Here's how the part is built. I have some questions about the finished solid (model axes, mm). A direction names the side the tool comes from. Coordinates: 2 decimals unless noted, no trailing zeros. Use a Markdown table: item, result. Add a question column.
Item 1: On a 3-axis mill with a long thin cutter (end or side, diameter ignored), from which of +Z, -Z, +X, -X, +Y, -Y can I reach the whole of each face in a straight line? I mean faces 5 (the cylindrical face through (3.04, -25.75, 0.06)), 6 (the conical face through (12.865, 0.153, -40.634)), 7 (the flat face through (7, 7, -30)), 8 (the flat face through (10, 15, -19)). Say none if no direction works.
Item 2: If we mould it in two halves opening along Z, with no side actions, what happens to faces 1 (the cylindrical face through (3.04, -0.12, -21.75)), 2 (the cylindrical face through (3.04, 25.75, -0.06)), 3 (the cylindrical face through (3.042, -19.696, 9.226)), 4 (the cylindrical face through (4.93, 12.25, -17.76))? For each: pulls with the +Z half, pulls with the -Z half, needs draft (parallel to the pull), parting line crosses it, or undercut.
Item 3: Imagine slicing it at A-A, the plane y = 0. Count the separate pieces of the cut face and the enclosed holes in it, and give its area (3 significant figures).
Item 4: If I drill on line 1 along Z through (x, y) = (6.75, -0.5); line 2 along Y through (x, z) = (4.75, 0); line 3 along X through (y, z) = (10, 22), over which ranges is the centre line in solid material (lowest first)? Write a range as from..to.
Item 5: Will these pins go through, and if not, where does the flat tip stop? pin 1 Ø9 at (y, z) = (-16, 18) entering from +X; pin 2 Ø10.5 at (y, z) = (0, -30) entering from +X; pin 3 Ø2.5 at (y, z) = (22, 0.5) entering from +X; pin 4 Ø9 at (y, z) = (0, -30) entering from -X.
```python
from build123d import *

# Parameters (mm, degrees)
SKETCH_1_R               = 26.5
SKETCH_1_R_2             = 16.5
EXTRUDE_1_DEPTH          = 6
SKETCH_2_R               = 2.05
CUT_EXTRUDE_1_DEPTH      = 10
PATTERN_CIRCULAR_1_COUNT = 3
PATTERN_CIRCULAR_1_ANGLE = 100
SKETCH_3_R               = 2.05
SKETCH_3_R_2             = 2.6
SKETCH_3_R_3             = 16.5
EXTRUDE_2_DEPTH          = 7
CUT_EXTRUDE_START        = -6
CUT_EXTRUDE_2_OUTLINE_R  = 26.5
CUT_EXTRUDE_2_DEPTH      = 6
CHAMFER_1_SIZE           = 1
FILLET_1_R               = 5
SKETCH_5_R               = 4.075
SKETCH_5_R_2             = 4
CUT_EXTRUDE_3_DEPTH      = 3
PATTERN_CIRCULAR_2_COUNT = 2
PATTERN_CIRCULAR_2_ANGLE = 50
F_2_THE_OTHER_WAY_COUNT  = 2
F_2_THE_OTHER_WAY_ANGLE  = 50
SKETCH_6_R               = 6.6
CUT_EXTRUDE_4_DEPTH      = 4
SKETCH_7_R               = 7.6
CUT_EXTRUDE_5_DEPTH      = 1
SKETCH_8_R               = 6.15
CUT_EXTRUDE_6_DEPTH      = 2
CHAMFER_2_SIZE           = 0.5


# Read off the part's stored shape, not the designer's step: 切除-拉伸2
with BuildPart() as part:
    # 草图1 → 凸台-拉伸1 (new body)
    with BuildSketch(Plane(origin=(0, 0, 0), x_dir=(0, 0, -1), z_dir=(1, 0, 0))):
        Circle(SKETCH_1_R)
        Circle(SKETCH_1_R_2, mode=Mode.SUBTRACT)
    extrude(amount=EXTRUDE_1_DEPTH)

    # 草图2 → 切除-拉伸1 (cut)
    with BuildSketch(Plane.ZY):
        with Locations((16.661466638, 13.980630511)):
            Circle(SKETCH_2_R)
        with Locations((-16.661466638, -13.980630511)):
            Circle(SKETCH_2_R)
    cut_extrude_1 = extrude(amount=-CUT_EXTRUDE_1_DEPTH, mode=Mode.SUBTRACT)

    # 阵列(圆周)1: 切除-拉伸1 ×3 about axis
    pattern_circular_1_axis = Axis((0, 0, 0), (-1, 0, 0))
    for i in range(1, PATTERN_CIRCULAR_1_COUNT):
        add(cut_extrude_1.rotate(pattern_circular_1_axis, i * PATTERN_CIRCULAR_1_ANGLE / (PATTERN_CIRCULAR_1_COUNT - 1)), mode=Mode.SUBTRACT)

    # 草图3 → 凸台-拉伸2 (add)
    with BuildSketch(Plane.ZY.offset(-6)):
        with BuildLine():
            ThreePointArc((-35.683333333, 9.418052995), (-41, 0), (-35.683333333, -9.418052995))
            Line((-35.683333333, -9.418052995), (-13.691666667, -22.688945852))
            ThreePointArc((-13.691666667, -22.688945852), (26.5, 0), (-13.691666667, 22.688945852))
            Line((-13.691666667, 22.688945852), (-35.683333333, 9.418052995))
        make_face()
        with Locations((-16.661466638, -13.980630511)):
            Circle(SKETCH_3_R, mode=Mode.SUBTRACT)
        with Locations(Location((0, -21.75, 0), (0, 0, 50))):
            Circle(SKETCH_3_R, mode=Mode.SUBTRACT)
        with Locations(Location((16.661466638, -13.980630511, 0), (0, 0, 100))):
            Circle(SKETCH_3_R, mode=Mode.SUBTRACT)
        with Locations(Location((-30, 0, 0), (0, 0, 180))):
            Circle(SKETCH_3_R_2, mode=Mode.SUBTRACT)
        with Locations(Location((-16.661466638, 13.980630511, 0), (0, 0, 100))):
            Circle(SKETCH_3_R, mode=Mode.SUBTRACT)
        with Locations(Location((0, 0, 0), (0, 0, 180))):
            Circle(SKETCH_3_R_3, mode=Mode.SUBTRACT)
        with Locations(Location((0, 21.75, 0), (0, 0, 50))):
            Circle(SKETCH_3_R, mode=Mode.SUBTRACT)
        with Locations((16.661466638, 13.980630511)):
            Circle(SKETCH_3_R, mode=Mode.SUBTRACT)
    extrude(amount=-EXTRUDE_2_DEPTH)

    # 切除-拉伸2 outline → 切除-拉伸2 (cut)
    with BuildSketch(Plane.ZY.offset(CUT_EXTRUDE_START)):
        Circle(CUT_EXTRUDE_2_OUTLINE_R)
        with BuildLine():
            ThreePointArc((-18.939960291, -10.693007255), (-21.75, 0), (-18.939960291, 10.693007255))
            ThreePointArc((-18.939960291, 10.693007255), (-19.72564441, 16.551780949), (-13.819446038, 16.795398513))
            ThreePointArc((-13.819446038, 16.795398513), (-9.191947193, 19.712194368), (-3.983053015, 21.382183908))
            ThreePointArc((-3.983053015, 21.382183908), (0, 25.75), (3.983053015, 21.382183908))
            ThreePointArc((3.983053015, 21.382183908), (9.191947193, 19.712194368), (13.819446038, 16.795398513))
            ThreePointArc((13.819446038, 16.795398513), (19.72564441, 16.551780949), (18.939960291, 10.693007255))
            ThreePointArc((18.939960291, 10.693007255), (21.75, 0), (18.939960291, -10.693007255))
            ThreePointArc((18.939960291, -10.693007255), (19.72564441, -16.551780949), (13.819446038, -16.795398513))
            ThreePointArc((13.819446038, -16.795398513), (9.191947193, -19.712194368), (3.983053015, -21.382183908))
            ThreePointArc((3.983053015, -21.382183908), (0, -25.75), (-3.983053015, -21.382183908))
            ThreePointArc((-3.983053015, -21.382183908), (-9.191947193, -19.712194368), (-13.819446038, -16.795398513))
            ThreePointArc((-13.819446038, -16.795398513), (-19.72564441, -16.551780949), (-18.939960291, -10.693007255))
        make_face(mode=Mode.SUBTRACT)
    extrude(amount=CUT_EXTRUDE_2_DEPTH, mode=Mode.SUBTRACT)

    # 倒角1
    chamfer_1_edges = [part.edges().sort_by_distance(p)[0] for p in [
        (13, 0, 16.5),
        (0, 0, 16.5),
    ]]
    chamfer(chamfer_1_edges, length=CHAMFER_1_SIZE)

    # 圆角1
    fillet_1_edges = [part.edges().sort_by_distance(p)[0] for p in [
        (3, 10.693007255, -18.939960291),
        (3, -10.693007255, -18.939960291),
        (3, -16.795398513, -13.819446038),
        (3, -21.382183908, -3.983053015),
        (3, -21.382183908, 3.983053015),
        (3, -16.795398513, 13.819446038),
        (3, -10.693007255, 18.939960291),
        (3, 10.693007255, 18.939960291),
        (3, 16.795398513, 13.819446038),
        (3, 21.382183908, 3.983053015),
        (3, 21.382183908, -3.983053015),
        (3, 16.795398513, -13.819446038),
    ]]
    fillet(fillet_1_edges, radius=FILLET_1_R)

    # 草图5 → 切除-拉伸3 (cut)
    with BuildSketch(Plane(origin=(13, 0, 0), x_dir=(0, 0, -1), z_dir=(1, 0, 0))):
        with Locations((0, 21.75)):
            Circle(SKETCH_5_R)
        with Locations((0, -21.75)):
            Circle(SKETCH_5_R_2)
    cut_extrude_3 = extrude(amount=-CUT_EXTRUDE_3_DEPTH, mode=Mode.SUBTRACT)

    # 阵列(圆周)2: 切除-拉伸3 ×2 about axis
    pattern_circular_2_axis = Axis((0, 0, 0), (-1, 0, 0))
    for i in range(1, PATTERN_CIRCULAR_2_COUNT):
        add(cut_extrude_3.rotate(pattern_circular_2_axis, i * PATTERN_CIRCULAR_2_ANGLE / (PATTERN_CIRCULAR_2_COUNT - 1)), mode=Mode.SUBTRACT)

    # 2 the other way: 切除-拉伸3 ×2 about axis
    f_2_the_other_way_axis = Axis((0, 0, 0), (1, 0, 0))
    for i in range(1, F_2_THE_OTHER_WAY_COUNT):
        add(cut_extrude_3.rotate(f_2_the_other_way_axis, i * F_2_THE_OTHER_WAY_ANGLE / (F_2_THE_OTHER_WAY_COUNT - 1)), mode=Mode.SUBTRACT)

    # 草图6 → 切除-拉伸4 (cut)
    with BuildSketch(Plane.ZY.offset(-6)):
        with Locations((-30, 0)):
            Circle(SKETCH_6_R)
    extrude(amount=-CUT_EXTRUDE_4_DEPTH, mode=Mode.SUBTRACT)

    # 草图7 → 切除-拉伸5 (cut)
    with BuildSketch(Plane.ZY.offset(-6)):
        with Locations((-30, 0)):
            Circle(SKETCH_7_R)
    extrude(amount=-CUT_EXTRUDE_5_DEPTH, mode=Mode.SUBTRACT)

    # 草图8 → 切除-拉伸6 (cut)
    with BuildSketch(Plane(origin=(13, 0, 0), x_dir=(0, 0, -1), z_dir=(1, 0, 0))):
        with Locations((30, 0)):
            Circle(SKETCH_8_R)
    extrude(amount=-CUT_EXTRUDE_6_DEPTH, mode=Mode.SUBTRACT)

    # 倒角2
    chamfer_2_edges = [part.edges().sort_by_distance(p)[0] for p in [
        (6, 16.053499424, -24.6875),
        (6, 0, -41),
        (13, 16.053499424, -24.6875),
        (6, -16.053499424, -24.6875),
        (13, 0, -41),
        (13, 0, 26.5),
        (13, -16.053499424, -24.6875),
        (6, 0, 26.5),
    ]]
    chamfer(chamfer_2_edges, length=CHAMFER_2_SIZE)


solid = part.part
```
Ans:
| question | item | result |
|---|---|---|
| 1 | face 5 | -X, -Y |
| 1 | face 6 | -Z, +X |
| 1 | face 7 | -X |
| 1 | face 8 | +X |
| 2 | face 1 | pulls with the -Z half |
| 2 | face 2 | parting line crosses it |
| 2 | face 3 | pulls with the +Z half |
| 2 | face 4 | undercut |
| 3 | separate pieces | 3 |
| 3 | enclosed holes | 0 |
| 3 | area | 217 mm^2 |
| 4 | line 1 | z = -40.99..-37.58, -22.42..-16.49, 16.49..26.5 |
| 4 | line 2 | y = -25.75..-23.8, -19.7..-16.5, 16.5..19.7, 23.8..25.75 |
| 4 | line 3 | x = 6..13 |
| 5 | pin 1 | stops at x = 13 |
| 5 | pin 2 | stops at x = 11 |
| 5 | pin 3 | passes through |
| 5 | pin 4 | stops at x = 10 |
